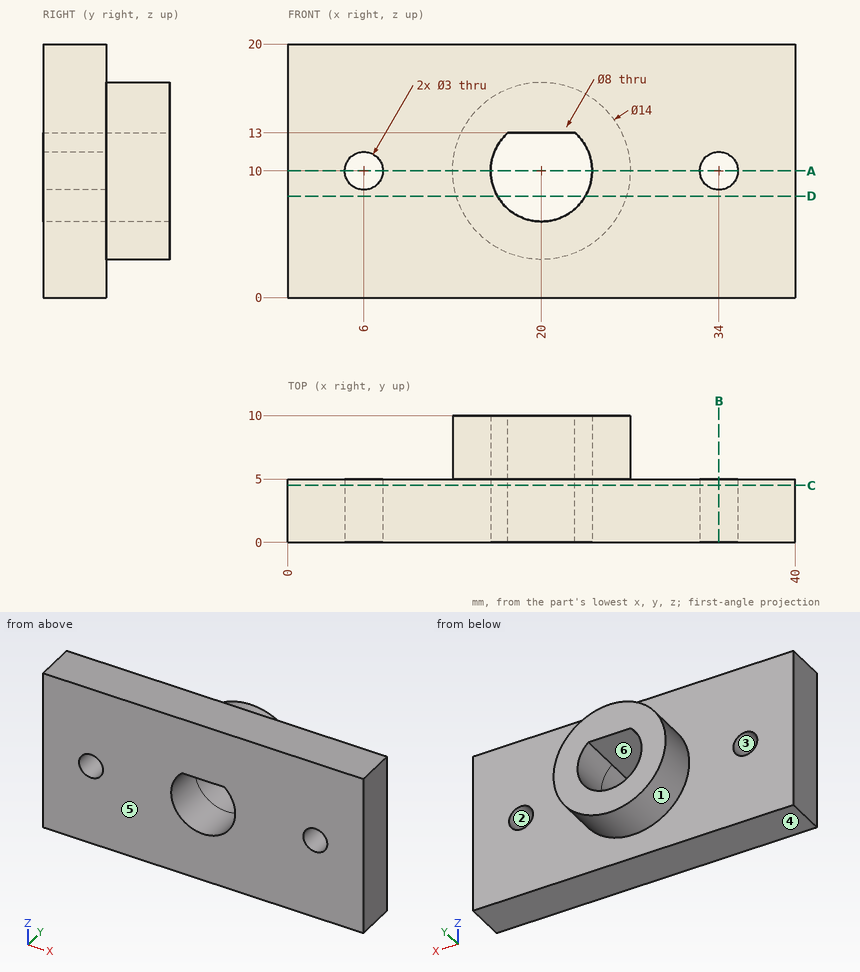
Study the drawing (mm; zero at the part's minimum x, y, z) and answer. A direction names the side the tool comes from. Round coordinates to 2 decimals unless told otherwise and drop trailing zeros. Write each loop counter-clockwise with the first axis right and the second up, starting at its lowest first coordinate (ties: lowest second). Pieces come first, ordered by that corner, then holes. Notation, with made-up numbers: (82.5, 5.25) - (97.5, 5.25) arc R27 cw to (97.5, 25.25) - close; hole circle Ø8 at (39, 52.5). An arc over 180 degrees is marked (long way). Use a Markdown table: item, result. Add a question column.
1. A tool of negligible diameter and unlimited length cuts with its end or side. For the marked faces 5 and 6, from which of +Z, -Z, +X, -X, +Y, -Y can it reach the whole face along a straight path? Write none if from no direction.
2. The part is cut by section C-C (y = 4.5). Write down the section's boundary in (x, z).
3. For a pull along Z with two mould halves and no side action, classify the marked faces 1, 2, 3 and 4 as +Z half, -Z half, draft (parallel to the pull), parting line (faces both ways), or undercut.
4. The part is cut by section B-B (x = 34). Write down the section's boundary in (y, z).
5. The part is cut by section A-A (z = 10). Write down the section's boundary in (x, y), and give its area (3 significant figures).
6. Flat-ended cylindrical pins translate along their axes: P1, Ø5, axis at x = 20, z = 10, coming from the +Y side; P2, Ø5, axis at x = 6, z = 10, coming from the +Y side; P3, Ø2, axis at y = 6.5, z = 12.5, coming from the +X side; P4, Ø2.5, axis at x = 19, y = 6.5, coming from the -Z side. Find the tip coordinate at first contact, or state that the pin passes through.
7. Consider line 1 (X direction, y = 3.1, z = 10); line 2 (X direction, y = 8.9, z = 10); line 3 (X direction, y = 1.25, z = 7). Determine where each line is inside the solid, lowest interval first.
8. The part is cut by section D-D (z = 8). Write down the section's boundary in (x, y), and give its area (3 significant figures).
Reported:
| question | item | result |
|---|---|---|
| 1 | face 5 | +Z, -Z, +X, -X, -Y |
| 1 | face 6 | +Y, -Y |
| 2 | outline | (0, 0) - (40, 0) - (40, 20) - (0, 20) - close; hole circle Ø3 at (6, 10); hole (17.35, 13) arc R4 ccw (long way) to (22.65, 13) - close; hole circle Ø3 at (34, 10) |
| 3 | face 1 | parting line |
| 3 | face 2 | undercut |
| 3 | face 3 | undercut |
| 3 | face 4 | -Z half |
| 4 | outline | (0, 0) - (5, 0) - (5, 8.5) - (0, 8.5) - close; (0, 11.5) - (5, 11.5) - (5, 20) - (0, 20) - close |
| 5 | outline | (0, 0) - (4.5, 0) - (4.5, 5) - (0, 5) - close; (7.5, 0) - (16, 0) - (16, 10) - (13, 10) - (13, 5) - (7.5, 5) - close; (24, 0) - (32.5, 0) - (32.5, 5) - (27, 5) - (27, 10) - (24, 10) - close; (35.5, 0) - (40, 0) - (40, 5) - (35.5, 5) - close |
| 5 | area | 160 mm^2 |
| 6 | P1 | through |
| 6 | P2 | y = 5 |
| 6 | P3 | x = 26.84 |
| 6 | P4 | z = 3 |
| 7 | line 1 | 0 to 4.5, 7.5 to 16, 24 to 32.5, 35.5 to 40 |
| 7 | line 2 | 13 to 16, 24 to 27 |
| 7 | line 3 | 0 to 17.35, 22.65 to 40 |
| 8 | outline | (0, 0) - (16.54, 0) - (16.54, 10) - (13.29, 10) - (13.29, 5) - (0, 5) - close; (23.46, 0) - (40, 0) - (40, 5) - (26.71, 5) - (26.71, 10) - (23.46, 10) - close |
| 8 | area | 198 mm^2 |
